from build123d import *

# Parameters (mm, degrees)
SKETCH1_W           = 60
SKETCH1_H           = 60
BOSS_EXTRUDE1_DEPTH = 5
SKETCH2_R           = 2
HOLE_DEPTH          = 5
SKETCH3_R           = 12
BOSS_EXTRUDE2_DEPTH = 8
SHAFT_DEPTH         = 20
SKETCH5_R           = 30
GEAR_DEPTH          = 30
SKETCH6_R           = 20
MOTOR_DEPTH         = 65


with BuildPart() as part:
    # Sketch1 → Boss-Extrude1 (new body)
    with BuildSketch(Plane.XY):
        Rectangle(SKETCH1_W, SKETCH1_H)
    extrude(amount=BOSS_EXTRUDE1_DEPTH)

    # Sketch2 → hole (cut)
    with BuildSketch(Plane(origin=(0, 0, 0), x_dir=(-1, 0, 0), z_dir=(0, 0, -1))):
        with Locations((-25, 25)):
            Circle(SKETCH2_R)
        with Locations((25, 25)):
            Circle(SKETCH2_R)
        with Locations((25, -25)):
            Circle(SKETCH2_R)
        with Locations((-25, -25)):
            Circle(SKETCH2_R)
    extrude(amount=-HOLE_DEPTH, mode=Mode.SUBTRACT)

    # Sketch3 → Boss-Extrude2 (add)
    with BuildSketch(Plane(origin=(0, 0, 0), x_dir=(-1, 0, 0), z_dir=(0, 0, -1))):
        Circle(SKETCH3_R)
    extrude(amount=-BOSS_EXTRUDE2_DEPTH)

    # Sketch4 → shaft (add)
    with BuildSketch(Plane.XY.offset(8)):
        with BuildLine():
            Line((-2.645751311, 3), (2.645751311, 3))
            ThreePointArc((2.645751311, 3), (0, -4), (-2.645751311, 3))
        make_face()
    extrude(amount=SHAFT_DEPTH)

    # Sketch5 → gear (add)
    with BuildSketch(Plane(origin=(0, 0, 0), x_dir=(-1, 0, 0), z_dir=(0, 0, -1))):
        Circle(SKETCH5_R)
    extrude(amount=GEAR_DEPTH)

    # Sketch6 → motor (add)
    with BuildSketch(Plane(origin=(0, 0, -30), x_dir=(-1, 0, 0), z_dir=(0, 0, -1))):
        Circle(SKETCH6_R)
    extrude(amount=MOTOR_DEPTH)


solid = part.part
Check sheet for the modelled part. Datum: model origin and axes. Units: mm. A direction names the side the tool comes from. Give positions to 0.01 mm unless a question says otherwise; leave off trailing zeros. Loops run counter-clockwise (first coordinate to the right, second up) from the corner with the lowest first, then second, coordinate; pieces in that order, holes last. Notation, with made-up numbers: M -37,-13 L -22,-13 A12 cw -22,-3 Z; hole C 41,-20.75 d4. An arc over 180 degrees is marked long. Answer as a JSON object with one key per item and string values. Group by question number.
Q1. Cross-section at D-D on y = 4.5. Record the cut outline in (x, z), then the cut area to 3 significant figures.
Q2. Material ranges on line 1 along Y through (x, z) = (-25, 2.9); line 2 along Z through (x, y) = (16, -14); line 3 along Z through (x, y) = (2, -17.5), recorded low to high. Write a range as [from, to].
Q3. Cross-section at B-B on y = 25. Record the cut outline in (x, z), then the cut area to 3 significant figures.
Q4. Cross-section at C-C on z = 12. Record the cut outline in (x, y).
Q5. Access from +Z, -Z, +X, -X, +Y, -Y to the whole of each face (thin tool, end or side, straight path). Record for faces 4 (the flat face through (-6, -20, -30)), 5 (the flat face through (-14, 0, 5)), 6 (the flat face through (-23, 24, 0)).
Q6. Go/stop test with flat-tipped pins: P1, Ø3, axis at x = 18.5, z = -25, coming from the +Y side; P2, Ø15, axis at x = -20, y = -22, coming from the -Z side; P3, Ø4, axis at x = 1, z = 21, coming from the +Y side; P4, Ø3.5, axis at x = 25, y = -25, coming from the -Z side. Record where each tip stops, or that it passes through.
Q7. Release check for a two-part mould opening along Y. For faces 1 (the cylindrical face through (-23.4, 23.8, 2.5)), 2 (the flat face through (23, 24, 0)), 3 (the cylindrical face through (29.97, 1.32, -14.79)) record: released by +Y, released by -Y, zero draft, split by the parting line, or undercut.
Q8. Cross-section at A-A on x = 24.5. Record the cut outline in (y, z), then the cut area to 3 significant figures.
Evaluation:
{
 "1": {"outline": "M -30,0 L -29.66,0 L -29.66,-30 L -19.49,-30 L -19.49,-95 L 19.49,-95 L 19.49,-30 L 29.66,-30 L 29.66,0 L 30,0 L 30,5 L 11.12,5 L 11.12,8 L -11.12,8 L -11.12,5 L -30,5 Z", "area": "4,680 mm2"},
 "2": {"line 1": "y = [-30, -27], [-23, 23], [27, 30]", "line 2": "z = [-30, 5]", "line 3": "z = [-95, 5]"},
 "3": {"outline": "M -30,0 L -27,0 L -27,5 L -30,5 Z; M -23,0 L -16.58,0 L -16.58,-30 L 16.58,-30 L 16.58,0 L 23,0 L 23,5 L -23,5 Z; M 27,0 L 30,0 L 30,5 L 27,5 Z", "area": "1,250 mm2"},
 "4": {"outline": "M -2.65,3 A4 ccw long 2.65,3 Z"},
 "5": {"face 4": "-Z", "face 5": "+Z", "face 6": "-Z, -X, +Y"},
 "6": {"P1": "stops at y = 24.72", "P2": "stops at z = -30", "P3": "stops at y = 3", "P4": "passes through"},
 "7": {"face 1": "undercut", "face 2": "zero draft", "face 3": "split by the parting line"},
 "8": {"outline": "M -30,0 L -26.94,0 L -26.94,5 L -30,5 Z; M -23.06,0 L -17.31,0 L -17.31,-30 L 17.31,-30 L 17.31,0 L 23.06,0 L 23.06,5 L -23.06,5 Z; M 26.94,0 L 30,0 L 30,5 L 26.94,5 Z", "area": "1,300 mm2"}
}
